Read the model definition and answer for the solid it produces. Units are mm, in the model's axes. Face numbers are marked on the shaded views. A direction names the side the tool comes from. Coordinates: 2 decimals unless noted, no trailing zeros. Write each loop counter-clockwise with the first axis right and the second up, starting at its lowest first coordinate (ties: lowest second). Pieces come first, ordered by that corner, then holes. Notation, with made-up numbers: M 1.5,-1 L 38.5,-1 A17 ccw 38.5,20 Z; hole C 82,68 d5. An arc over 180 degrees is marked long. Write item = value, one per line.
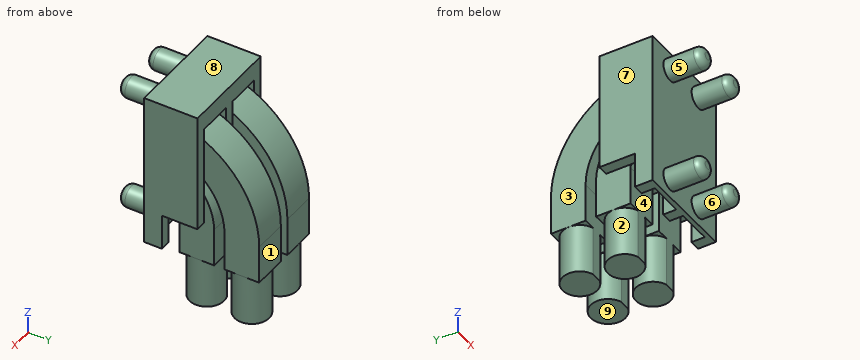
from build123d import *

# Parameters (mm, degrees)
SZKIC1_W                    = 5.7
SZKIC1_H                    = 8.7
DODANIE_WYCI_GNI_CIE1_DEPTH = 3
SZKIC5_W                    = 1.95
SZKIC5_H                    = 7.65
WYTNIJ_WYCI_GNI_CIE2_DEPTH  = 2.75
SZKIC3_W                    = 2
SZKIC3_H                    = 2
WYTNIJ_WYCI_GNI_CIE1_DEPTH  = 9.802840451
SZKIC6_R                    = 0.6
DODANIE_WYCI_GNI_CIE2_DEPTH = 2.1
ZAOKR_GLENIE1_R             = 0.4
DODANIE_WYCI_GNI_CIE3_DEPTH = 1.95
DODANIE_WYCI_GNI_CIE4_DEPTH = 1.95
SZKIC9_OUTSIDE_W            = 10.8
SZKIC9_OUTSIDE_H            = 13.3
SZKIC9_OUTSIDE_R            = 0.975
WYTNIJ_WYCI_GNI_CIE4_DEPTH  = 2.8


with BuildPart() as part:
    # Szkic1 → Dodanie-wyciągnięcie1 (new body)
    with BuildSketch(Plane(origin=(0, 0, 0), x_dir=(1, 0, 0), z_dir=(0, 1, 0))):
        Rectangle(SZKIC1_W, SZKIC1_H)
    extrude(amount=DODANIE_WYCI_GNI_CIE1_DEPTH)

    # Szkic5 → Wytnij-wyciągnięcie2 (cut)
    with BuildSketch(Plane(origin=(0, 3, 0), x_dir=(1, 0, 0), z_dir=(0, 1, 0))):
        with Locations((1.27, 0.525)):
            Rectangle(SZKIC5_W, SZKIC5_H)
        with Locations((-1.27, 0.525)):
            Rectangle(SZKIC5_W, SZKIC5_H)
    extrude(amount=-WYTNIJ_WYCI_GNI_CIE2_DEPTH, mode=Mode.SUBTRACT)

    # Szkic3 → Wytnij-wyciągnięcie1 (cut, through all)
    with BuildSketch(Plane(origin=(2.85, 0, 1.65), x_dir=(0, 0, 1), z_dir=(-1, 0, 0))):
        with Locations((-5, 2)):
            Rectangle(SZKIC3_W, SZKIC3_H)
    extrude(amount=WYTNIJ_WYCI_GNI_CIE1_DEPTH, mode=Mode.SUBTRACT)

    # Szkic6 → Dodanie-wyciągnięcie2 (add)
    with BuildSketch(Plane.XZ):
        with Locations(Location((1.27, 3.3, 0), (0, 0, 90))):
            Circle(SZKIC6_R)
        with Locations(Location((-1.27, 3.3, 0), (0, 0, 90))):
            Circle(SZKIC6_R)
        with Locations(Location((1.27, -3.3, 0), (0, 0, 90))):
            Circle(SZKIC6_R)
        with Locations(Location((-1.27, -3.3, 0), (0, 0, 90))):
            Circle(SZKIC6_R)
    extrude(amount=DODANIE_WYCI_GNI_CIE2_DEPTH)

    # Zaokrąglenie1
    zaokr_glenie1_edges = [part.edges().sort_by_distance(p)[0] for p in [
        (1.27, -2.1, 2.7),
        (-1.27, -2.1, 2.7),
        (1.27, -2.1, -3.9),
        (-1.27, -2.1, -3.9),
    ]]
    fillet(zaokr_glenie1_edges, radius=ZAOKR_GLENIE1_R)

    # Szkic7 → Dodanie-wyciągnięcie3 (add)
    with BuildSketch(Plane(origin=(0.295, 0, 0), x_dir=(0, 0, -1), z_dir=(1, 0, 0))):
        with BuildLine():
            Line((2.55, 6.1), (7.5, 6.1))
            Line((7.5, 6.1), (7.5, 4.15))
            Line((7.5, 4.15), (2.55, 4.15))
            ThreePointArc((2.55, 4.15), (-0.207716447, 3.007716447), (-1.35, 0.25))
            Line((-1.35, 0.25), (-3.3, 0.25))
            ThreePointArc((-3.3, 0.25), (-1.58657467, 4.38657467), (2.55, 6.1))
        make_face()
    dodanie_wyci_gni_cie3 = extrude(amount=DODANIE_WYCI_GNI_CIE3_DEPTH)

    # Szkic8 → Dodanie-wyciągnięcie4 (add)
    with BuildSketch(Plane(origin=(0.295, 0, 0), x_dir=(0, 0, -1), z_dir=(1, 0, 0))):
        with BuildLine():
            Line((7.5, 3.56), (2.55, 3.56))
            ThreePointArc((2.55, 3.56), (0.209476554, 2.590523446), (-0.76, 0.25))
            Line((-0.76, 0.25), (1.19, 0.25))
            ThreePointArc((1.19, 0.25), (1.588334778, 1.211665222), (2.55, 1.61))
            Line((2.55, 1.61), (7.5, 1.61))
            Line((7.5, 1.61), (7.5, 3.56))
        make_face()
    dodanie_wyci_gni_cie4 = extrude(amount=DODANIE_WYCI_GNI_CIE4_DEPTH)

    # Lustro2: Dodanie-wyciągnięcie3, Dodanie-wyciągnięcie4 across plane
    add(dodanie_wyci_gni_cie3.mirror(Plane.ZY))
    add(dodanie_wyci_gni_cie4.mirror(Plane.ZY))

    # Szkic9 outside → Wytnij-wyciągnięcie4 (cut)
    with BuildSketch(Plane(origin=(0, 0, -7.5), x_dir=(-1, 0, 0), z_dir=(0, 0, -1))):
        with Locations((0, 2)):
            Rectangle(SZKIC9_OUTSIDE_W, SZKIC9_OUTSIDE_H)
        with Locations((-1.27, 2.54)):
            Circle(SZKIC9_OUTSIDE_R, mode=Mode.SUBTRACT)
        with Locations((-1.27, 5.08)):
            Circle(SZKIC9_OUTSIDE_R, mode=Mode.SUBTRACT)
        with Locations((1.27, 5.08)):
            Circle(SZKIC9_OUTSIDE_R, mode=Mode.SUBTRACT)
        with Locations((1.27, 2.54)):
            Circle(SZKIC9_OUTSIDE_R, mode=Mode.SUBTRACT)
    extrude(amount=-WYTNIJ_WYCI_GNI_CIE4_DEPTH, mode=Mode.SUBTRACT)


solid = part.part
Item 1: Find section C-C (x = 0.1). Determine the outline of the cut face in (y, z), and give its area (3 significant figures).
Worked answers:
outline = M 0,-4.35 L 1,-4.35 L 1,-2.35 L 3,-2.35 L 3,4.35 L 0,4.35 Z
area = 22.1 mm²
Item 2: Which of the six approach directions +Z, -Z, +X, -X, +Y, -Y give full straight-line access (tool end or side, diameter ignored) to the marked faces 1, 2, 3, 4 and 5?
Worked answers:
face_1 = +Z, -Z, +X, -X, +Y
face_2 = -Z
face_3 = +Z, -Z, -X, +Y
face_4 = -Z, +X, -X
face_5 = -Y
Item 3: For a pull along Z with two mould halves and no side action, classify the marked faces 6, 7, 8 and 9 as released by +Z, released by -Z, zero draft, split by the parting line, or undercut.
Worked answers:
face_6 = undercut
face_7 = zero draft
face_8 = released by +Z
face_9 = released by -Z
Item 4: Flat-ended cylindrical pins translate along their axes: pin 1 (1.5 mm diameter, centred on x = 2, z = 2, fed in from -Y); pin 2 (2 mm diameter, centred on y = 3, z = -2.5, fed in from -X); pin 3 (0.7 mm diameter, centred on x = 2.5, y = 1.5, fed in from -Z); pin 4 (0.6 mm diameter, centred on x = -1.5, z = 1, fed in from +Y). Find the tip coordinate at first contact, or state that the pin passes through.
Worked answers:
pin_1 = 0
pin_2 = -2.85
pin_3 = -4.7
pin_4 = 5.11
Item 5: Find section B-B (z = -0.5). Determine the outline of the cut face in (x, y) (3 decimals).
Worked answers:
outline = M -2.85,0 L 2.85,0 L 2.85,3 L 2.245,3 L 2.245,2.849 L 0.295,2.849 L 0.295,3 L -0.295,3 L -0.295,2.849 L -2.245,2.849 L -2.245,3 L -2.85,3 Z; M -2.245,3.568 L -0.295,3.568 L -0.295,5.729 L -2.245,5.729 Z; M 0.295,3.568 L 2.245,3.568 L 2.245,5.729 L 0.295,5.729 Z
Item 6: Consider line 1 along Y through (x, z) = (0.6, -3.75); line 2 along X through (y, z) = (5.75, -3.5) (3 decimals); line 3 along Y through (x, z) = (-0.1, -1.5). Determine where each line is inside the solid, lowest interval first. Write a range as from..to.
Worked answers:
line_1 = 0..0.25, 1.61..3.56, 4.15..6.1
line_2 = -2.245..-0.295, 0.295..2.245
line_3 = 0..3
Item 7: Find section D-D (y = 4.5). Determine the outline of the cut face in (x, z) (3 decimals).
Worked answers:
outline = M -2.245,-4.7 L -2.054,-4.7 L -2.054,-7.5 L -0.486,-7.5 L -0.486,-4.7 L -0.295,-4.7 L -0.295,1.47 L -2.245,1.47 Z; M 0.295,-4.7 L 0.486,-4.7 L 0.486,-7.5 L 2.054,-7.5 L 2.054,-4.7 L 2.245,-4.7 L 2.245,1.47 L 0.295,1.47 Z
Item 8: Find section A-A (z = -6.25). Determine the outline of the cut face in (x, y) (3 decimals), and give its area (3 significant figures).
Worked answers:
outline = M -1.563,1.61 L -0.977,1.61 A0.975 ccw long Z; M -1.563,4.15 L -0.977,4.15 A0.975 ccw long Z; M 0.977,1.61 L 1.563,1.61 A0.975 ccw long Z; M 0.977,4.15 L 1.563,4.15 A0.975 ccw long Z
area = 11.9 mm²
